Verification items for the finished model (mm, model axes). A direction names the side the tool comes from. Coordinates: 2 decimals unless noted, no trailing zeros. Loops run counter-clockwise (first coordinate to the right, second up) from the corner with the lowest first, then second, coordinate; pieces in that order, holes last. Notation, with made-up numbers: (-5.75, -30) - (29.25, -30) arc R18 ccw to (29.25, -7) - close; hole circle Ø10 at (-4.5, 57). An arc over 180 degrees is marked (long way). One line per item, written item: value. Start each with the question number.
(1) Section check A-A (z = 68.75). Record the boundary of the cut face in (x, y).
(2) Section check B-B (x = 72). Record the boundary of the cut face in (y, z).
(3) Draft check along X on faces 3 (the face through (120, 5, 2)), 4 (the face through (-120, 5, 2)), 5 (the face through (85, 5, 1)), 6 (the face through (-2, 0, 105)). Enter one of: +X half, -X half, draft (parallel to the pull), parting line (faces both ways), or undercut.
(4) Section check D-D (x = 0). Record the boundary of the cut face in (y, z), plus the area to 3 significant figures.
(5) Set-up check for faces 1 (the face through (-1, 5, 85)), 2 (the face through (0.392, 7.812, 98.264)): record each of +Z, -Z, +X, -X, +Y, -Y from which the full face is reachable in a straight line by a thin tool's end or side.
(6) Section check C-C (y = 5.25). Count the separate pieces of the cut face and the enclosed holes in it, plus the area to 3 significant figures.
(7) Thickness scan on probe 1 along X at (y, z) = (2.25, -25); probe 2 along X at (y, z) = (3.25, 68.75); probe 3 along Z at (x, y) = (-71, 7.25). Record the ranges inside material, lowest first. Write a range as [from, to].
```python
from build123d import *

# Parameters (mm, degrees)
SKETCH1_W                                       = 240
SKETCH1_H                                       = 240
BOSS_EXTRUDE1_DEPTH                             = 10
CSK_FOR_M5_FLAT_HEAD_MACHINE_SCREW1_D           = 5.8
CSK_FOR_M5_FLAT_HEAD_MACHINE_SCREW1_CSINK_D     = 10.4
CSK_FOR_M5_FLAT_HEAD_MACHINE_SCREW1_CSINK_ANGLE = 90
FILLET1_R                                       = 5
TAP_DRILL_FOR_M10X1_25_TAP1_D                   = 8.8
TAP_DRILL_FOR_M10X1_25_TAP1_DEPTH               = 19.75
TAP_DRILL_FOR_M10X1_25_TAP1_TIP                 = 2.643786724
SKETCH8_W                                       = 170
SKETCH8_H                                       = 170
CUT_EXTRUDE1_DEPTH                              = 10
FILLET2_R                                       = 5


with BuildPart() as part:
    # Sketch1 → Boss-Extrude1 (new body)
    with BuildSketch(Plane(origin=(0, 0, 0), x_dir=(1, 0, 0), z_dir=(0, 1, 0))):
        Rectangle(SKETCH1_W, SKETCH1_H)
    extrude(amount=BOSS_EXTRUDE1_DEPTH)

    # CSK for M5 Flat Head Machine Screw1 (through all)
    with Locations(Plane(origin=(0, 10, 0), x_dir=(1, 0, 0), z_dir=(0, 1, 0))):
        with Locations((-111.25, 68.75), (0, 101.25), (111.25, 68.75), (111.25, -68.75), (0, -101.25), (-111.25, -68.75)):
            CounterSinkHole(CSK_FOR_M5_FLAT_HEAD_MACHINE_SCREW1_D / 2, CSK_FOR_M5_FLAT_HEAD_MACHINE_SCREW1_CSINK_D / 2, counter_sink_angle=CSK_FOR_M5_FLAT_HEAD_MACHINE_SCREW1_CSINK_ANGLE)

    # Fillet1
    fillet1_edges = [part.edges().sort_by_distance(p)[0] for p in [
        (120, 5, 120),
        (-120, 5, 120),
        (-120, 5, -120),
        (120, 5, -120),
    ]]
    fillet(fillet1_edges, radius=FILLET1_R)

    # Tap Drill for M10x1.25 Tap1
    with Locations(Plane(origin=(0, 10, 0), x_dir=(1, 0, 0), z_dir=(0, 1, 0))):
        with Locations((107.5, 25), (-107.5, 25)):
            Hole(TAP_DRILL_FOR_M10X1_25_TAP1_D / 2, depth=TAP_DRILL_FOR_M10X1_25_TAP1_DEPTH)
            with Locations((0, 0, -(TAP_DRILL_FOR_M10X1_25_TAP1_DEPTH + TAP_DRILL_FOR_M10X1_25_TAP1_TIP / 2))):  # 118° drill point
                Cone(0, TAP_DRILL_FOR_M10X1_25_TAP1_D / 2, TAP_DRILL_FOR_M10X1_25_TAP1_TIP, mode=Mode.SUBTRACT)

    # Sketch8 → Cut-Extrude1 (cut)
    with BuildSketch(Plane(origin=(0, 10, 0), x_dir=(1, 0, 0), z_dir=(0, 1, 0))):
        Rectangle(SKETCH8_W, SKETCH8_H)
    extrude(amount=-CUT_EXTRUDE1_DEPTH, mode=Mode.SUBTRACT)

    # Fillet2
    fillet2_edges = [part.edges().sort_by_distance(p)[0] for p in [
        (-85, 5, -85),
        (85, 5, -85),
        (85, 5, 85),
        (-85, 5, 85),
    ]]
    fillet(fillet2_edges, radius=FILLET2_R)


solid = part.part
```
Responses:
1. outline: (-120, 0) - (-114.15, 0) - (-114.15, 7.7) - (-116.45, 10) - (-120, 10) - close; (-108.35, 0) - (-85, 0) - (-85, 10) - (-106.05, 10) - (-108.35, 7.7) - close; (85, 0) - (108.35, 0) - (108.35, 7.7) - (106.05, 10) - (85, 10) - close; (114.15, 0) - (120, 0) - (120, 10) - (116.45, 10) - (114.15, 7.7) - close
2. outline: (0, -120) - (10, -120) - (10, -85) - (0, -85) - close; (0, 85) - (10, 85) - (10, 120) - (0, 120) - close
3. face 3: +X half
3. face 4: -X half
3. face 5: undercut
3. face 6: draft
4. outline: (0, -120) - (10, -120) - (10, -106.45) - (7.7, -104.15) - (0, -104.15) - close; (0, -98.35) - (7.7, -98.35) - (10, -96.05) - (10, -85) - (0, -85) - close; (0, 85) - (10, 85) - (10, 96.05) - (7.7, 98.35) - (0, 98.35) - close; (0, 104.15) - (7.7, 104.15) - (10, 106.45) - (10, 120) - (0, 120) - close
4. area: 573 mm²
5. face 1: +Y, -Y
5. face 2: +Y
6. separate pieces: 1
6. enclosed holes: 9
6. area: 28,400 mm²
7. probe 1: x = [-120, -111.9], [-103.1, -85], [85, 103.1], [111.9, 120]
7. probe 2: x = [-120, -114.15], [-108.35, -85], [85, 108.35], [114.15, 120]
7. probe 3: z = [-120, -85], [85, 120]
